Design review of the part built by this model. Coordinates are the model's own, in mm. A direction names the side the tool comes from. Coordinates: 2 decimals unless noted, no trailing zeros. Write each loop counter-clockwise with the first axis right and the second up, starting at its lowest first coordinate (ties: lowest second). Pieces come first, ordered by that corner, then holes. Notation, with made-up numbers: (25, -4) -> (65, -4) arc R23 ccw to (65, 26) -> close; hole circle Ø3 at (89.5, 18). An arc over 180 degrees is marked (long way). Answer in a Markdown table with one row per item. Add a question column.
Item 1: For faces 1 (the face through (-8, -8, -26)), 2 (the face through (-8, 0, -26)), list the 3-axis set-ups (+Z, -Z, +X, -X, +Y, -Y) from which the entire face can be reached by the end or side of a thin tool; tool diameter is ignored.
Item 2: Clearance check with flat-ended pins moving along their axes: P1, Ø10, axis at x = 390, y = 24, coming from the -Z side; P2, Ø8, axis at x = 174, z = -22, coming from the +Y side. State where each tip first meets the part, or that it passes through.
Item 3: Take a section at C-C, the plane y = 25. Write out the cut boundary in (x, z).
Item 4: Take a section at B-B, the plane z = -22.5. Write out the cut boundary in (x, y).
Item 5: To check wall thickness, follow line 1 (Y direction, x = -116.5, z = -29); line 2 (Z direction, x = 368, y = 26); line 3 (Z direction, x = -497.5, y = 27.5). State the ranges of each line that lie inside material, in increasing order.
Item 6: Take a section at A-A, the plane x = 227.5. Write out the cut boundary in (y, z), and give its area (3 significant figures).
from build123d import *

# Parameters (mm, degrees)
SKETCH2_W            = 1200
SKETCH2_H            = 40
BASE_FLANGE1_DEPTH   = 8
EDGE_FLANGE1_START   = -600
EDGE_FLANGE1_DEPTH   = 1200
EDGE_FLANGE1_2_DEPTH = 1200


# Read off the part's stored shape, not the designer's step: Edge-Flange1
# Sheet-metal steps are written as plain solids
with BuildPart() as part:
    # Sketch2 → Base-Flange1 (new body)
    with BuildSketch(Plane(origin=(0, 0, 0), x_dir=(1, 0, 0), z_dir=(0, 1, 0))):
        with Locations((0, 20)):
            Rectangle(SKETCH2_W, SKETCH2_H)
    extrude(amount=-BASE_FLANGE1_DEPTH)

    # Edge-Flange1 outline → Edge-Flange1 (cut)
    with BuildSketch(Plane.YZ.offset(EDGE_FLANGE1_START)):
        with BuildLine():
            ThreePointArc((-8, -10.77542358), (-6.328529058, -4.946311673), (-1.822082615, -0.88868907))
            Line((-1.822082615, -0.88868907), (0, 0))
            Line((0, 0), (-8, 0))
            Line((-8, 0), (-8, -10.77542358))
        make_face()
    extrude(amount=EDGE_FLANGE1_DEPTH, mode=Mode.SUBTRACT)

    # Edge-Flange1 2 outline → Edge-Flange1 2 (add)
    with BuildSketch(Plane.YZ.offset(EDGE_FLANGE1_START)):
        with BuildLine():
            Line((35.142114222, 17.139954337), (0, 0))
            Line((0, 0), (0, -10.77542358))
            ThreePointArc((0, -10.77542358), (0.455855712, -9.185665787), (1.68488656, -8.079041441))
            Line((1.68488656, -8.079041441), (38.649083397, 9.949601967))
            Line((38.649083397, 9.949601967), (35.142114222, 17.139954337))
        make_face()
    extrude(amount=EDGE_FLANGE1_2_DEPTH)


solid = part.part
Answers:
| question | item | result |
|---|---|---|
| 1 | face 1 | +Z, -Z, +X, -X, -Y |
| 1 | face 2 | -Z, +X, -X, +Y |
| 2 | P1 | stops at z = 0.37 |
| 2 | P2 | stops at y = 0 |
| 3 | outline | (-600, 3.29) -> (600, 3.29) -> (600, 12.19) -> (-600, 12.19) -> close |
| 4 | outline | (-600, -8) -> (600, -8) -> (600, 0) -> (-600, 0) -> close |
| 5 | line 1 | y = -8 to 0 |
| 5 | line 2 | z = 3.78 to 12.68 |
| 5 | line 3 | z = 4.51 to 13.41 |
| 6 | outline | (-8, -40) -> (0, -40) -> (0, -10.78) arc R3 cw to (1.68, -8.08) -> (38.65, 9.95) -> (35.14, 17.14) -> (-1.82, -0.89) arc R11 ccw to (-8, -10.78) -> close |
| 6 | area | 625 mm^2 |
